Model file for the job. Use its own axes, mm. A direction names the side the tool comes from. Coordinates: 2 decimals unless noted, no trailing zeros. Write each loop counter-clockwise with the first axis right and the second up, starting at its lowest first coordinate (ties: lowest second). Pieces come first, ordered by that corner, then holes.
Q1. Which spindle directions (+Z, -Z, +X, -X, +Y, -Y) get a long thin tool onto all of the face, cutting with end or side? Do faces 1 (the flat face through (12, -11.38, 4)), 2 (the cylindrical face through (2.12, -10.45, 5.58)). Say none if no direction does.
Q2. Band-saw the part on D-D, the plane x = 13.5. Write the cut outline in (y, z).
Q3. Band-saw the part on B-B, the plane z = 3. Write the cut outline in (x, y).
Q4. Band-saw the part on A-A, the plane x = 8.5. Write the cut outline in (y, z).
Q5. Band-saw the part on C-C, the plane y = -10.25. Write the cut outline in (x, z) (3 decimals).
Q6. Pull direction Z, two halves, no side cores. Call faces 3 (the cylindrical face through (1.477, -10.452, 11.983)), 4 (the flat face through (4, -11.38, 4)), 5 (the flat face through (8, -5, 15.8)): released by +Z, released by -Z, zero draft, split by the parting line, or undercut.
Q7. Drill centre lines: probe 1 along Y at (x, z) = (8.75, 4.25); probe 2 along Z at (x, y) = (12.5, -10.5); probe 3 along X at (y, z) = (-10.5, 3.75). Where is each one in solid material? Low to high.
from build123d import *

# Parameters (mm, degrees)
F0_W     = 15.8
F0_H     = 15.8
F1_DEPTH = 9.55
F2_R     = 2.45
F4_DEPTH = 1.83
F3_R     = 2.45
F6_DEPTH = 1.83
F7_R     = 0.1


with BuildPart() as f1:
    # F0 (on Front) → F1 (new body)
    with BuildSketch(Plane.XZ):
        with Locations((7.9, 7.9)):
            Rectangle(F0_W, F0_H)
    extrude(amount=F1_DEPTH)

    # F2 (on face) → F4 (join)
    with BuildSketch(Plane.XZ.offset(9.55)):
        with Locations((3.925, 11.875)):
            Circle(F2_R)
    extrude(amount=F4_DEPTH)

    # F3 (on face) → F6 (join)
    with BuildSketch(Plane.XZ.offset(9.55)):
        with Locations((11.875, 11.875)):
            Circle(F3_R)
        with Locations((3.925, 3.925)):
            Circle(F3_R)
        with Locations((11.875, 3.925)):
            Circle(F3_R)
    extrude(amount=F6_DEPTH)

    # F7
    f7_edges = [f1.edges().sort_by_distance(p)[0] for p in [
        (7.9, 0, 15.8),
        (0, 0, 7.9),
        (7.9, 0, 0),
        (15.8, 0, 7.9),
    ]]
    fillet(f7_edges, radius=F7_R)


solid = f1.part
Answer sheet:
1. face 1: +Z, -Z, +X, -X, -Y
1. face 2: -Y
2. outline: (-11.38, 2.09) - (-9.55, 2.09) - (-9.55, 0) - (-0.1, 0) arc R0.1 ccw to (0, 0.1) - (0, 15.7) arc R0.1 ccw to (-0.1, 15.8) - (-9.55, 15.8) - (-9.55, 13.71) - (-11.38, 13.71) - (-11.38, 10.04) - (-9.55, 10.04) - (-9.55, 5.76) - (-11.38, 5.76) - close
3. outline: (0, -9.55) - (1.66, -9.55) - (1.66, -11.38) - (6.19, -11.38) - (6.19, -9.55) - (9.61, -9.55) - (9.61, -11.38) - (14.14, -11.38) - (14.14, -9.55) - (15.8, -9.55) - (15.8, -0.1) arc R0.1 ccw to (15.7, 0) - (0.1, 0) arc R0.1 ccw to (0, -0.1) - close
4. outline: (-9.55, 0) - (-0.1, 0) arc R0.1 ccw to (0, 0.1) - (0, 15.7) arc R0.1 ccw to (-0.1, 15.8) - (-9.55, 15.8) - close
5. outline: circle Ø4.9 at (3.925, 3.925); circle Ø4.9 at (3.925, 11.875); circle Ø4.9 at (11.875, 3.925); circle Ø4.9 at (11.875, 11.875)
6. face 3: undercut
6. face 4: zero draft
6. face 5: released by +Z
7. probe 1: y = -9.55 to 0
7. probe 2: z = 1.56 to 6.29, 9.51 to 14.24
7. probe 3: x = 1.48 to 6.37, 9.43 to 14.32
